from build123d import *

# Parameters (mm, degrees)
SKETCH016_R     = 29.334526
PAD012_DEPTH    = 3
PAD013_DEPTH    = 15
CHAMFER001_SIZE = 1
FILLET009_R     = 1
FILLET010_R     = 3


with BuildPart() as part:
    # Sketch016 (on DatumPlane) → Pad012 (new body)
    with BuildSketch(Plane(origin=(-153.083157, 155.978406, 843), x_dir=(0, 1, 0), z_dir=(0, 0, 1))):
        Circle(SKETCH016_R)
    extrude(amount=PAD012_DEPTH)

    # Sketch017 (on Face3 of Pad012) → Pad013 (join)
    with BuildSketch(Plane(origin=(-153.083157, 155.978406, 846), x_dir=(0, 1, 0), z_dir=(0, 0, 1))):
        with BuildLine():
            ThreePointArc((-20.899311, 5.287957), (-26.187268, 0), (-20.899311, -5.287957))
            Line((-20.899311, -5.287957), (20.899313, -5.287957))
            ThreePointArc((20.899313, -5.287957), (26.18727, 0), (20.899313, 5.287957))
            Line((-20.899311, 5.287957), (20.899313, 5.287957))
        make_face()
    extrude(amount=PAD013_DEPTH)

    # Chamfer001
    chamfer001_edges = [part.edges().sort_by_distance(p)[0] for p in [
        (-153.083157, 126.64388, 846),
    ]]
    chamfer(chamfer001_edges, length=CHAMFER001_SIZE)

    # Fillet009
    fillet009_edges = [part.edges().sort_by_distance(p)[0] for p in [
        (-147.7952, 155.978406, 846),
    ]]
    fillet(fillet009_edges, radius=FILLET009_R)

    # Fillet010
    fillet010_edges = [part.edges().sort_by_distance(p)[0] for p in [
        (-147.7952, 155.978406, 861),
    ]]
    fillet(fillet010_edges, radius=FILLET010_R)


solid = part.part
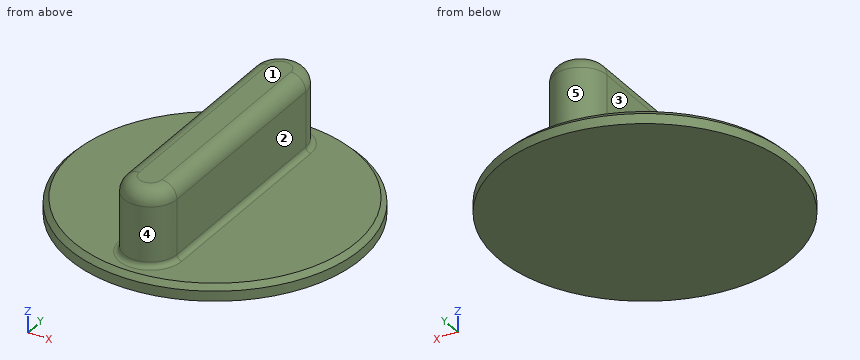
Build history of the part. All positions in model axes, mm. Face numbers are marked on the shaded views. A direction names the side the tool comes from. Round coordinates to 2 decimals unless told otherwise and drop trailing zeros. Use CSV: the item, a comma, the result in double quotes.
1. Wall check: probe 1 along Z at (x, y) = (-135, 157.5); probe 2 along X at (y, z) = (140, 855.5); probe 3 along X at (y, z) = (134.5, 849.75). Give the ranges that are in metal, low to high. Write a range as from..to.
Reply:
probe 1,"z = 843..846"
probe 2,"x = -158.37..-147.8"
probe 3,"x = -158.34..-147.83"
2. Flat gauge pins, fed straight in: pin 1 (8 mm diameter, centred on x = -144, z = 848, fed in from +Y); pin 2 (5 mm diameter, centred on y = 163.5, z = 859, fed in from +X); pin 3 (9 mm diameter, centred on y = 165, z = 851, fed in from +X). Where does each tip first touch, or does it go through?
Reply:
pin 1,"stops at y = 184.6"
pin 2,"stops at x = -147.8"
pin 3,"stops at x = -147.66"
3. Tool access for the marked faces 1, 2, 3, 4 and 5: list every direction of +Z, -Z, +X, -X, +Y, -Y with a clear straight run to the whole face (end or side of a thin tool).
Reply:
face 1,"+Z, +X, -X, +Y, -Y"
face 2,"+Z, +X, +Y, -Y"
face 3,"+Z, -X, +Y, -Y"
face 4,"+Z, -Y"
face 5,"+Z, +Y"
